from build123d import *

# Parameters (mm, degrees)
EXTRUDE_1_DEPTH = 6
EXTRUDE_2_DEPTH = 6
EXTRUDE_3_DEPTH = 6
SKETCH_4_R      = 1.5
EXTRUDE_4_DEPTH = 1.8
SKETCH_5_R      = 1.1
EXTRUDE_5_DEPTH = 10
EXTRUDE_6_DEPTH = 6


with BuildPart() as part:
    # Sketch 1 → Extrude 1 (new body)
    with BuildSketch(Plane.XY):
        Polygon((0, 10), (0, -10), (43.391858736, -36.953542991), (71.115712236, -22.772903722), (107.439932669, -22.772903722), (113.022851841, -17.18998455), (113.022851841, -14.359848661), (105.70299447, -14.359848661), (102.364936039, -17.697907092), (63.844827478, -17.697907092), (43.391858736, -28.159518127), (15.650074222, -10.927267577), (15.650074222, 10.927267577), (43.391858736, 28.159518127), (63.844827478, 17.697907092), (102.364936039, 17.697907092), (105.70299447, 14.359848661), (113.022851841, 14.359848661), (113.022851841, 17.18998455), (107.439932669, 22.772903722), (71.115712236, 22.772903722), (43.391858736, 36.953542991), align=None)
    extrude(amount=EXTRUDE_1_DEPTH)

    # Sketch 2 → Extrude 2 (add)
    with BuildSketch(Plane.XY.offset(6)):
        Polygon((113.022851841, 14.359848661), (111.256497416, 14.359848661), (112.311790012, 13.419299654), align=None)
        Polygon((111.256497416, 14.359848661), (109.362923156, 14.359848661), (110.418215751, 13.419299654), align=None)
        Polygon((109.362923156, 14.359848661), (107.584092484, 14.359848661), (108.52464149, 13.419299654), align=None)
        Polygon((107.584092484, 14.359848661), (105.70299447, 14.359848661), (106.643543477, 13.419299654), align=None)
        Polygon((105.70299447, -14.359848661), (107.584092484, -14.359848661), (106.643543477, -13.419299654), align=None)
        Polygon((107.584092484, -14.359848661), (109.362923156, -14.359848661), (108.52464149, -13.419299654), align=None)
        Polygon((109.362923156, -14.359848661), (111.256497416, -14.359848661), (110.418215751, -13.419299654), align=None)
        Polygon((111.256497416, -14.359848661), (113.022851841, -14.359848661), (112.311790012, -13.419299654), align=None)
    extrude(amount=-EXTRUDE_2_DEPTH)

    # Sketch 3 → Extrude 3 (add)
    with BuildSketch(Plane.XY.offset(6)):
        Polygon((26.69644411, 17.788895872), (44.940516172, 10.497320184), (61.640798283, 23.261107226), (62.960793136, 21.534011156), (46.260511025, 8.770224115), (46.260511025, -8.770224115), (62.960793136, -21.534011156), (61.640798283, -23.261107226), (44.940516172, -10.497320184), (26.69644411, -17.788895872), (15.650074222, -10.927267577), (15.650074222, 10.927267577), align=None)
    extrude(amount=-EXTRUDE_3_DEPTH)

    # Sketch 4 → Extrude 4 (add)
    with BuildSketch(Plane.ZY):
        with BuildLine():
            Line((-5.1, -10), (11.1, -10))
            ThreePointArc((11.1, -10), (12.514213562, -9.414213562), (13.1, -8))
            Line((13.1, -8), (13.1, 8))
            ThreePointArc((13.1, 8), (12.514213562, 9.414213562), (11.1, 10))
            Line((11.1, 10), (-5.1, 10))
            ThreePointArc((-5.1, 10), (-6.514213562, 9.414213562), (-7.1, 8))
            Line((-7.1, 8), (-7.1, -8))
            ThreePointArc((-7.1, -8), (-6.514213562, -9.414213562), (-5.1, -10))
        make_face()
        with Locations(Location((9.25, 0, 0), (0, 0, 270))):
            Circle(SKETCH_4_R, mode=Mode.SUBTRACT)
        with Locations(Location((-3.25, 0, 0), (0, 0, 270))):
            Circle(SKETCH_4_R, mode=Mode.SUBTRACT)
    extrude(amount=EXTRUDE_4_DEPTH)

    # Sketch 5 → Extrude 5 (add)
    with BuildSketch(Plane.XY.offset(6)):
        with Locations(Location((17.984736969, 0, 0), (0, 0, 180))):
            Circle(SKETCH_5_R)
        with Locations(Location((7.984736969, 0, 0), (0, 0, 180))):
            Circle(SKETCH_5_R)
        with Locations((7.984736969, -49.1)):
            Circle(SKETCH_5_R)
        with Locations((17.984736969, -49.1)):
            Circle(SKETCH_5_R)
    extrude(amount=EXTRUDE_5_DEPTH)


with BuildPart() as extrude_5_piece_1:
    # of the separate pieces the step leaves, piece 1, a body of its own (extrude_5_pieces)
    add(part.part.solids().sort_by_distance((0, -10, -5.1))[0])



with BuildPart() as extrude_5_piece_2:
    # of the separate pieces the step leaves, piece 2, a body of its own (extrude_5_pieces)
    add(part.part.solids().sort_by_distance((9.084736969, -49.1, 6))[0])


with BuildPart() as extrude_5_piece_3:
    # of the separate pieces the step leaves, piece 3, a body of its own (extrude_5_pieces)
    add(part.part.solids().sort_by_distance((19.084736969, -49.1, 6))[0])


with BuildPart() as extrude_5_piece_1_1:
    add(extrude_5_piece_1.part)

    add(extrude_5_piece_2.part)  # Extrude 6 merges Extrude 5 piece 2

    add(extrude_5_piece_3.part)  # Extrude 6 merges Extrude 5 piece 3
    # Sketch 6 → Extrude 6 (add)
    with BuildSketch(Plane(origin=(0, 0, 6), x_dir=(-1, 0, 0), z_dir=(0, 0, -1))):
        Polygon((-15.984736969, -19.929173528), (-19.984736969, -22.413837129), (-19.984736969, -51.1), (-5.984736969, -51.1), (-5.984736969, -13.717514526), (-9.984736969, -16.202178127), (-9.984736969, -47.1), (-15.984736969, -47.1), align=None)
    extrude(amount=EXTRUDE_6_DEPTH)


solid = extrude_5_piece_1_1.part
Work out the finished part from the listing and answer in its coordinate system (mm). A direction names the side the tool comes from. Round coordinates to 2 decimals unless told otherwise and drop trailing zeros. Write each loop counter-clockwise with the first axis right and the second up, starting at its lowest first coordinate (ties: lowest second). Pieces come first, ordered by that corner, then holes. Notation, with made-up numbers: (41.5, 46.5) - (46.5, 46.5) arc R10 cw to (46.5, 62.5) - close; hole circle Ø7 at (11, 6.25). An arc over 180 degrees is marked (long way). Answer in a Markdown table with one row per item. Add a question column.
1. A cutting plane is placed at A-A, the plane z = -3.25. Determine the outline of the cut face in (x, y).
2. The mould has two halves that part along X. Classify faces 4 (the flat face through (83, 17.698, 3)), 5 (the flat face through (113.023, -16, 3)), 6 (the flat face through (40, 0, 0)): +X half, -X half, draft (parallel to the pull), parting line (faces both ways), or undercut.
3. For faces 1 (the flat face through (104.534, -15.529, 2.958)), 2 (the cylindrical face through (7.746, -50.174, 10.93)), 3 (the flat face through (57.448, 29.764, 2.958)), determine the directions among +Z, -Z, +X, -X, +Y, -Y from which every point of the face is accessible in a straight line to the end or side of a thin tool.
4. Given pin 1 (10 mm diameter, centred on x = 36, z = 10, fed in from +Y); pin 2 (5 mm diameter, centred on y = 0, z = 9.25, fed in from +X); pin 3 (5 mm diameter, centred on y = -43.5, z = 4, fed in from +X), each flat-ended and moving along its own axis, determine where each tip first touches the part or whether it passes through.
5. A cutting plane is placed at D-D, the plane y = -31. Determine the outline of the cut face in (x, z), and give its area (3 significant figures).
6. A cutting plane is placed at C-C, the plane x = 53. Determine the outline of the cut face in (y, z) (3 decimals), and give its area (3 significant figures).
7. Find the intervals of material crossed by line 1 along Z through (x, y) = (-0.75, 0); line 2 along Y through (x, z) = (78, 0.5); line 3 along X through (y, z) = (-19, 4), in increasing order. Write a range as from..to.
8. A cutting plane is placed at B-B, the plane x = 76.5. Determine the outline of the cut face in (y, z), and give its area (3 significant figures).
Worked out:
| question | item | result |
|---|---|---|
| 1 | outline | (-1.8, -10) - (0, -10) - (0, -1.5) - (-1.8, -1.5) - close; (-1.8, 1.5) - (0, 1.5) - (0, 10) - (-1.8, 10) - close |
| 2 | face 4 | undercut |
| 2 | face 5 | +X half |
| 2 | face 6 | draft |
| 3 | face 1 | +Z, -Z |
| 3 | face 2 | +Z |
| 3 | face 3 | +Z, -Z, +X, +Y |
| 4 | pin 1 | y = 34.23 |
| 4 | pin 2 | x = 19.08 |
| 4 | pin 3 | x = 19.98 |
| 5 | outline | (5.98, 0) - (9.98, 0) - (9.98, 6) - (5.98, 6) - close; (15.98, 0) - (19.98, 0) - (19.98, 6) - (15.98, 6) - close; (33.81, 0) - (55.03, 0) - (55.03, 6) - (33.81, 6) - close |
| 5 | area | 175 mm^2 |
| 6 | outline | (-32.039, 0) - (-23.245, 0) - (-23.245, 6) - (-32.039, 6) - close; (-16.657, 0) - (-13.921, 0) - (-13.921, 6) - (-16.657, 6) - close; (13.921, 0) - (16.657, 0) - (16.657, 6) - (13.921, 6) - close; (23.245, 0) - (32.039, 0) - (32.039, 6) - (23.245, 6) - close |
| 6 | area | 138 mm^2 |
| 7 | line 1 | -7.1..-4.75, -1.75..7.75, 10.75..13.1 |
| 7 | line 2 | -22.77..-17.7, 17.7..22.77 |
| 7 | line 3 | 5.98..9.98, 14.49..28.65, 56.07..59.65, 61.3..111.21 |
| 8 | outline | (-22.77, 0) - (-17.7, 0) - (-17.7, 6) - (-22.77, 6) - close; (17.7, 0) - (22.77, 0) - (22.77, 6) - (17.7, 6) - close |
| 8 | area | 60.9 mm^2 |
